Read the model definition and answer for the solid it produces. Units are mm, in the model's axes. Face numbers are marked on the shaded views. A direction names the side the tool comes from. Coordinates: 2 decimals unless noted, no trailing zeros. Order: outer loops, then holes, each group sorted by start corner. A loop starts at its lowest first (then second) coordinate and runs counter-clockwise, first axis right, second up.
```python
from build123d import *

# Parameters (mm, degrees)
F0_W      = 88.9
F0_H      = 66.675
F1_DEPTH  = 3.175
F2_W      = 88.9
F2_H      = 66.675
F2_W_2    = 82.55
F2_H_2    = 60.325
F3_DEPTH  = 19.05
F4_R      = 2.54
F5_DEPTH  = 4.7625
F6_R      = 1.397
F1_FACE_W = 82.55
F1_FACE_H = 60.325
F1_FACE_R = 2.54
F10_DEPTH = 2.54
F7_R      = 1.397
F11_DEPTH = 2.54
F8_R      = 1.397
F12_DEPTH = 2.54
F9_R      = 1.397
F13_DEPTH = 2.54
F14_W     = 9.652
F14_H     = 12.6365
F15_DEPTH = 3.175
F14_W_2   = 12.7
F16_DEPTH = 3.175
F18_DEPTH = 1.5875
F19_W     = 1.5875000006
F19_H     = 18.288
F20_DEPTH = 1.5875
F21_SIZE  = 2.54
F22_SIZE  = 2.54
F23_SIZE  = 2.54


with BuildPart() as f1:
    # F0 (on Top) → F1 (new body)
    with BuildSketch(Plane.XY):
        with Locations((44.45, 33.3375)):
            Rectangle(F0_W, F0_H)
    extrude(amount=F1_DEPTH)

    # F2 (on face) → F3 (join)
    with BuildSketch(Plane.XY.offset(3.175)):
        with Locations((44.45, 33.3375)):
            Rectangle(F2_W, F2_H)
        with Locations((44.45, 33.3375)):
            Rectangle(F2_W_2, F2_H_2, mode=Mode.SUBTRACT)
    extrude(amount=F3_DEPTH)

    # F4 (on face) → F5 (join)
    with BuildSketch(Plane.XY.offset(3.175)):
        with Locations((17.145, 57.3237927139)):
            Circle(F4_R)
        with Locations((17.145, 9.2075)):
            Circle(F4_R)
        with Locations((67.945, 42.2275)):
            Circle(F4_R)
        with Locations((67.945, 14.2875)):
            Circle(F4_R)
    extrude(amount=F5_DEPTH)

    # F6 (on face) + F1_face (on face) → F10 (join)
    with BuildSketch(Plane.XY.offset(7.9375)):
        with Locations((17.145, 57.3237927139)):
            Circle(F6_R)
    with BuildSketch(Plane(origin=(44.45, 33.3375, 3.175), x_dir=(1, 0, 0), z_dir=(0, 0, 1))):
        Rectangle(F1_FACE_W, F1_FACE_H)
        with Locations((-27.305, -24.13)):
            Circle(F1_FACE_R, mode=Mode.SUBTRACT)
        with Locations((23.495, -19.05)):
            Circle(F1_FACE_R, mode=Mode.SUBTRACT)
        with Locations((-27.305, 23.9862927139)):
            Circle(F1_FACE_R, mode=Mode.SUBTRACT)
        with Locations((23.495, 8.89)):
            Circle(F1_FACE_R, mode=Mode.SUBTRACT)
    extrude(amount=F10_DEPTH)

    # F7 (on face) → F11 (join)
    with BuildSketch(Plane.XY.offset(7.9375)):
        with Locations((67.945, 42.2275)):
            Circle(F7_R)
    extrude(amount=F11_DEPTH)

    # F8 (on face) → F12 (join)
    with BuildSketch(Plane.XY.offset(7.9375)):
        with Locations((17.145, 9.2075)):
            Circle(F8_R)
    extrude(amount=F12_DEPTH)

    # F9 (on face) → F13 (join)
    with BuildSketch(Plane.XY.offset(7.9375)):
        with Locations((67.945, 14.2875)):
            Circle(F9_R)
    extrude(amount=F13_DEPTH)

    # F14 (on face) → F15 (cut, through all)
    with BuildSketch(Plane(origin=(0, 0, 0), x_dir=(0, -1, 0), z_dir=(-1, 0, 0))):
        with Locations((-16.9198646352, 15.90675)):
            Rectangle(F14_W, F14_H)
    extrude(amount=-F15_DEPTH, mode=Mode.SUBTRACT)

    # F14 (on face) → F16 (cut, through all)
    with BuildSketch(Plane(origin=(0, 0, 0), x_dir=(0, -1, 0), z_dir=(-1, 0, 0))):
        with Locations((-46.3838646352, 15.90675)):
            Rectangle(F14_W_2, F14_H)
    extrude(amount=-F16_DEPTH, mode=Mode.SUBTRACT)

    # F17 (on face) → F18 (join)
    with BuildSketch(Plane.XY.offset(22.225)):
        Polygon((87.3125, 1.5875), (1.5875, 1.5875), (1.5875, 12.0938646352), (0, 12.0938646352), (0, 0), (88.9, 0), (88.9, 66.675), (0, 66.675), (0, 52.7338646352), (1.5875, 52.7338646352), (1.5875, 65.0875), (87.3125, 65.0875), align=None)
    extrude(amount=F18_DEPTH)

    # F19 (on face) → F20 (join)
    with BuildSketch(Plane.XY.offset(22.225)):
        with Locations((0.7937500003, 30.8898646352)):
            Rectangle(F19_W, F19_H)
    extrude(amount=F20_DEPTH)

    # F21
    f21_edges = [f1.edges().sort_by_distance(p)[0] for p in [
        (88.9, 0, 11.90625),
        (0, 0, 11.90625),
        (88.9, 66.675, 11.90625),
        (0, 66.675, 11.90625),
    ]]
    chamfer(f21_edges, length=F21_SIZE)

    # F22
    f22_edges = [f1.edges().sort_by_distance(p)[0] for p in [
        (3.175, 63.5, 13.97),
        (85.725, 63.5, 13.97),
        (85.725, 3.175, 13.97),
        (3.175, 3.175, 13.97),
    ]]
    chamfer(f22_edges, length=F22_SIZE)

    # F23 (call 1 of 4: OpenCascade refuses the feature's edges together)
    f23_edges = [f1.edges().sort_by_distance(p)[0] for p in [
        (44.45, 0, 0),
    ]]
    chamfer(f23_edges, length=F23_SIZE)

    # F23#2 (call 2 of 4)
    f23_2_edges = [f1.edges().sort_by_distance(p)[0] for p in [
        (88.9, 33.3375, 0),
    ]]
    chamfer(f23_2_edges, length=F23_SIZE)

    # F23#3 (call 3 of 4)
    f23_3_edges = [f1.edges().sort_by_distance(p)[0] for p in [
        (44.45, 66.675, 0),
    ]]
    chamfer(f23_3_edges, length=F23_SIZE)

    # F23#4 (call 4 of 4)
    f23_4_edges = [f1.edges().sort_by_distance(p)[0] for p in [
        (0, 33.3375, 0),
    ]]
    chamfer(f23_4_edges, length=F23_SIZE)


solid = f1.part
```
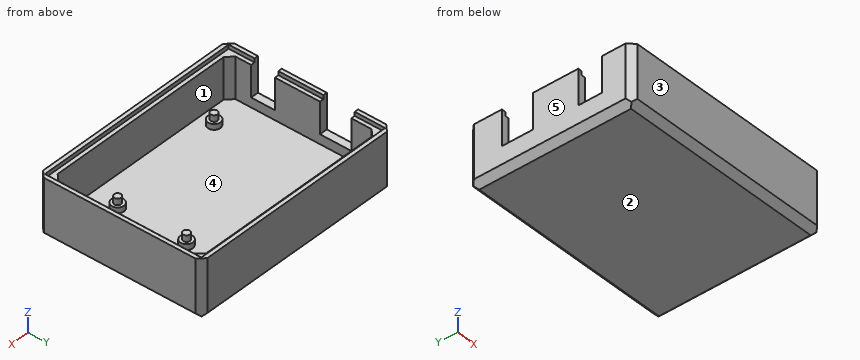
1) Which of the six approach directions +Z, -Z, +X, -X, +Y, -Y give full straight-line access (tool end or side, diameter ignored) to the marked faces 1 and 2?
A:
face 1: +Z
face 2: -Z, +X, -X, +Y, -Y
2) A cutting plane is placed at A-A, the plane z = 19.25. Determine the outline of the cut face in (x, y) (3 decimals).
A:
outline: (0, 2.54) - (2.54, 0) - (86.36, 0) - (88.9, 2.54) - (88.9, 64.135) - (86.36, 66.675) - (2.54, 66.675) - (0, 64.135) - (0, 52.734) - (3.175, 52.734) - (3.175, 60.96) - (5.715, 63.5) - (83.185, 63.5) - (85.725, 60.96) - (85.725, 5.715) - (83.185, 3.175) - (5.715, 3.175) - (3.175, 5.715) - (3.175, 12.094) - (0, 12.094) - close; (0, 21.746) - (3.175, 21.746) - (3.175, 40.034) - (0, 40.034) - close
3) Flat-ended cylindrical pins translate along their axes: pin 1 Ø8 at (x, y) = (54.5, 43) entering from +Z (3 decimals); pin 2 Ø3.5 at (x, y) = (2, 47.5) entering from +Z; pin 3 Ø2 at (x, y) = (17, 57.5) entering from +Z; pin 4 Ø0.5 at (y, z) = (39.5, 23.5) entering from -X. Find the tip coordinate at first contact, or state that the pin passes through.
A:
pin 1: stops at z = 5.715
pin 2: stops at z = 9.59
pin 3: stops at z = 10.48
pin 4: stops at x = 0
4) A cutting plane is placed at D-D, the plane y = 49. Determine the outline of the cut face in (x, z) (1 decimal), and give its area (3 significant figures).
A:
outline: (0, 2.5) - (2.5, 0) - (86.4, 0) - (88.9, 2.5) - (88.9, 23.8) - (87.3, 23.8) - (87.3, 22.2) - (85.7, 22.2) - (85.7, 5.7) - (3.2, 5.7) - (3.2, 9.6) - (0, 9.6) - close
area: 569 mm2
5) Straight lines are drawn through the part: line 1 (Y direction, x = 65, z = 8.75) (3 decimals); line 2 (X direction, y = 24, z = 12.5) (3 decimals); line 3 (Z direction, x = 32.5, y = 55) (3 decimals). For each, find the intervals that lie inside material, in ascending order.
A:
line 1: y = 0 to 3.175, 63.5 to 66.675
line 2: x = 0 to 3.175, 85.725 to 88.9
line 3: z = 0 to 5.715
6) A cutting plane is placed at B-B, the plane y = 36.5. Determine the outline of the cut face in (x, z) (1 decimal), and give its area (3 significant figures).
A:
outline: (0, 2.5) - (2.5, 0) - (86.4, 0) - (88.9, 2.5) - (88.9, 23.8) - (87.3, 23.8) - (87.3, 22.2) - (85.7, 22.2) - (85.7, 5.7) - (3.2, 5.7) - (3.2, 22.2) - (1.6, 22.2) - (1.6, 23.8) - (0, 23.8) - close
area: 611 mm2
7) A cutting plane is placed at C-C, the plane x = 62. Determine the outline of the cut face in (y, z) (1 decimal).
A:
outline: (0, 2.5) - (2.5, 0) - (64.1, 0) - (66.7, 2.5) - (66.7, 23.8) - (65.1, 23.8) - (65.1, 22.2) - (63.5, 22.2) - (63.5, 5.7) - (3.2, 5.7) - (3.2, 22.2) - (1.6, 22.2) - (1.6, 23.8) - (0, 23.8) - close
8) Determine the mould class of the marked faces 3, 4 and 5 for opening direction Y: pulls with the +Y half, pulls with the -Y half, needs draft (parallel to the pull), parting line crosses it, or undercut.
A:
face 3: pulls with the -Y half
face 4: undercut
face 5: needs draft
